from build123d import *

# Parameters (mm, degrees)
F1_DEPTH    = 30
F2_R        = 6.5
F3_DEPTH    = 30
F4_R        = 10
F5_DEPTH    = 12
F6_R        = 10
F7_DEPTH    = 12
F8_SIZE     = 3
F9_T2_ANGLE = 227.2231239027
F9_T4_ANGLE = 227.2231239027


# Not quite as in the source:
# - a fillet or chamfer that OpenCascade refuses, or shapes differently, is made with other operations: its cross-section is extruded or revolved along the edge and cut away or added


with BuildPart() as f1:
    # F0 (on Top) → F1 (new body)
    with BuildSketch(Plane.XY):
        with BuildLine():
            Line((30, 0), (60, 0))
            ThreePointArc((60, 0), (0, 60), (-60, 0))
            Line((-60, 0), (-30, 0))
            ThreePointArc((-30, 0), (0, 30), (30, 0))
        make_face()
    extrude(amount=-F1_DEPTH)

    # F2 (on face) → F3 (cut, through all)
    with BuildSketch(Plane.XY):
        with Locations((20, 43)):
            Circle(F2_R)
        with Locations((-20, 43)):
            Circle(F2_R)
    extrude(amount=-F3_DEPTH, mode=Mode.SUBTRACT)

    # F4 (on face) → F5 (cut)
    with BuildSketch(Plane.XY):
        with Locations((20, 43)):
            Circle(F4_R)
        with Locations((-20, 43)):
            Circle(F4_R)
    extrude(amount=-F5_DEPTH, mode=Mode.SUBTRACT)

    # F6 (on face) → F7 (cut)
    with BuildSketch(Plane(origin=(0, 0, -30), x_dir=(1, 0, 0), z_dir=(0, 0, -1))):
        with Locations((-20, -43)):
            Circle(F6_R)
        with Locations((20, -43)):
            Circle(F6_R)
    extrude(amount=-F7_DEPTH, mode=Mode.SUBTRACT)

    # F8
    f8_edges = [f1.edges().sort_by_distance(p)[0] for p in [
        (0, 30, -30),
        (0, 30, 0),
    ]]
    chamfer(f8_edges, length=F8_SIZE)

    # F9: fillet of radius 12 on 2 edges, made by hand

    # F9_s1 → F9_t2 (revolve, cut)
    with BuildSketch(Plane(origin=(0, 0, 0), x_dir=(0, 0, 1), z_dir=(0.400533941, -0.9162819228, 0))):
        with BuildLine():
            ThreePointArc((-22.0627460668, 30), (-26.3053867539, 30.7750278397), (-30, 33))
            Line((-30, 33), (-27, 30))
            Line((-27, 30), (-22.0627460668, 30))
        make_face()
    revolve(axis=Axis((0, 0, -27), (0, 0, -1)), revolution_arc=F9_T2_ANGLE, mode=Mode.SUBTRACT)

    # F9_s3 → F9_t4 (revolve, cut)
    with BuildSketch(Plane(origin=(0, 0, 0), x_dir=(0, 0, 1), z_dir=(0.400533941, -0.9162819228, 0))):
        with BuildLine():
            ThreePointArc((-7.9372539332, 30), (-3.6946132461, 30.7750278397), (0, 33))
            Line((0, 33), (-3, 30))
            Line((-3, 30), (-7.9372539332, 30))
        make_face()
    revolve(axis=Axis((0, 0, -3), (0, 0, -1)), revolution_arc=F9_T4_ANGLE, mode=Mode.SUBTRACT)


solid = f1.part
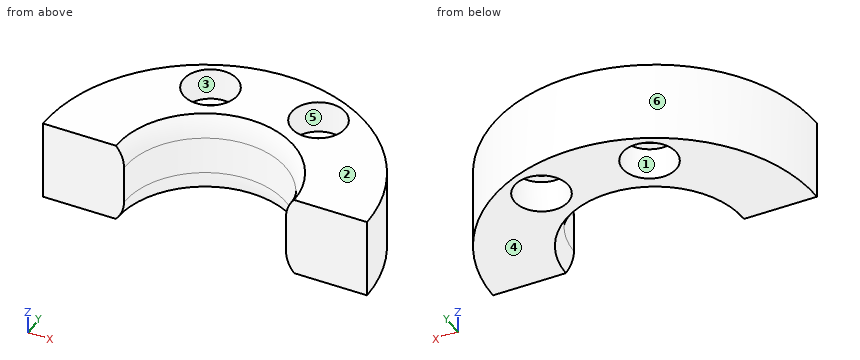
Verification items for the finished model (mm, model axes). Face numbers are marked on the shaded views. A direction names the side the tool comes from. Give positions to 0.01 mm unless a question says otherwise; leave off trailing zeros. Write each loop counter-clockwise with the first axis right and the second up, starting at its lowest first coordinate (ties: lowest second). Pieces come first, ordered by that corner, then holes. Notation, with made-up numbers: M 15.25,17.5 L 41.25,17.5 A14 cw 41.25,39.5 Z; hole C 80.5,47.5 d4. An arc over 180 degrees is marked long. Put each result on its own line as item: value. Start each with the question number.
1. Section check D-D (z = -26). Record the cut outline in (x, y).
2. Draft check along X on the marked faces 4, 5 and 6. Enter one of: +X half, -X half, draft (parallel to the pull), parting line (faces both ways), or undercut.
3. Scan lines: line 1 along Y through (x, z) = (18, -20.5); line 2 along Y through (x, z) = (-16.5, -10.5); line 3 along X through (y, z) = (42.5, -25.5). Record each from-to range of solid material in increasing order. Write a range as [from, to].
4. Section check C-C (y = 43). Record the cut outline in (x, z), and give its area (3 significant figures).
5. Section check A-A (z = -16). Record the cut outline in (x, y), and give its area (3 significant figures).
6. Set-up check for the marked faces 1, 2 and 3: record each of +Z, -Z, +X, -X, +Y, -Y from which the full face is reachable in a straight line by a thin tool's end or side.
7. Go/stop test with flat-tipped pins: pin 1 Ø12 at (x, y) = (39, 32.5) entering from +Z; pin 2 Ø3 at (y, z) = (17, -21) entering from +X; pin 3 Ø4 at (y, z) = (23.5, -17) entering from -X; pin 4 Ø6 at (x, z) = (4, -6.5) entering from -Y. Record where each tip stops, or that it passes through.
8. Section check B-B (x = 0). Record the cut outline in (y, z).
Answer list:
1. outline: M -60,0 L -30.66,0 A30.66 cw 30.66,0 L 60,0 A60 ccw Z; hole C -20,43 d20; hole C 20,43 d20
2. face 4: draft
2. face 5: undercut
2. face 6: parting line
3. line 1: [24, 33.2], [52.8, 57.24]
3. line 2: [25.05, 33.63], [52.37, 57.69]
3. line 3: [-42.35, -29.99], [-10.01, 10.01], [29.99, 42.35]
4. outline: M -41.84,-30 L -30,-30 L -30,-18 L -26.5,-18 L -26.5,-12 L -30,-12 L -30,0 L -41.84,0 Z; M -13.5,-18 L -10,-18 L -10,-30 L 10,-30 L 10,-18 L 13.5,-18 L 13.5,-12 L 10,-12 L 10,0 L -10,0 L -10,-12 L -13.5,-12 Z; M 26.5,-18 L 30,-18 L 30,-30 L 41.84,-30 L 41.84,0 L 30,0 L 30,-12 L 26.5,-12 Z
4. area: 1,390 mm2
5. outline: M -60,0 L -30,0 A30 cw 30,0 L 60,0 A60 ccw Z; hole C -20,43 d13; hole C 20,43 d13
5. area: 3,980 mm2
6. face 1: -Z
6. face 2: +Z, +X, -X, +Y, -Y
6. face 3: +Z
7. pin 1: z = 0
7. pin 2: x = 57.96
7. pin 3: x = -56.02
7. pin 4: y = 29.21
8. outline: M 30,-22.06 A12 ccw 33,-30 L 60,-30 L 60,0 L 33,0 A12 ccw 30,-7.94 Z
